The listing builds one solid part. Answer for the finished solid, in the listing's coordinates (mm). Face numbers are marked on the shaded views. A direction names the side the tool comes from. Round coordinates to 2 decimals unless told otherwise and drop trailing zeros. Write each loop counter-clockwise with the first axis right and the second up, starting at its lowest first coordinate (ties: lowest second). Pieces come first, ordered by that corner, then holes. Notation, with made-up numbers: M 3.5,-39 L 13.5,-39 A6 ccw 13.5,-31 Z; hole C 16.5,79 d9. An arc over 180 degrees is marked long. One line per item, written item: value. Start each with the question number.
(1) Given P1, Ø12, axis at x = -8, z = 12.5, coming from the -Y side; P2, Ø9.5, axis at x = 33.26, y = 5, coming from the +Z side; P3, Ø8, axis at x = 27, y = 7.5, coming from the +Z side, each flat-ended and moving along its own axis, determine where each tip first touches the part or whether it passes through.
(2) Section A-A (y = -12.5) is taken. Determine the outline of the cut face in (x, z) (3 decimals), plus the area to 3 significant figures.
(3) Section D-D (z = 16.5) is taken. Determine the outline of the cut face in (x, y) (3 decimals), plus the area to 3 significant figures.
(4) Section B-B (y = 5) is taken. State how many separate pieces and enclosed holes the cut face has, plus the area to 3 significant figures.
(5) Section C-C (x = -9) is taken. Determine the outline of the cut face in (y, z), plus the area to 3 significant figures.
(6) Consider probe 1 along X at (y, z) = (1.5, 6); probe 2 along X at (y, z) = (-21, 4) (3 decimals); probe 3 along Z at (x, y) = (-55, -12.5). Determine where each line is inside the solid, lowest interval first.
(7) For the marked faces 1, 2, 3 and 4, determine the directions among +Z, -Z, +X, -X, +Y, -Y from which every point of the face is accessible in a straight line to the end or side of a thin tool.
(8) For a pull along Z with two mould halves and no side action, classify the marked faces 5, 6 and 7 as released by +Z, released by -Z, zero draft, split by the parting line, or undercut.
Autodesk Inventor part; units mm, degrees
ref_plane "YZ Plane" through (0, 0, 0) normal (1, 0, 0) x (0, 1, 0)
ref_plane "XZ Plane" through (0, 0, 0) normal (0, 1, 0) x (-1, 0, 0)
ref_plane "XY Plane" through (0, 0, 0) normal (0, 0, 1) x (1, 0, 0)
sketch "Sketch1" plane through (0, 0, 0) normal (0, 1, 0) x (-1, 0, 0)
  line L0 (-15, 15) -> (15, 15)
  line L1 (15, 15) -> (15, -15)
  line L2 (15, -15) -> (-15, -15)
  line L3 (-15, 15) -> (15, -15) construction
  line L4 (15, 15) -> (-15, -15) construction
  line L5 (25, 25) -> (-25, 25)
  line L6 (-25, -25) -> (25, -25)
  line L7 (25, 25) -> (59.45, 25)
  line L8 (59.45, 25) -> (59.45, -25)
  line L9 (59.45, -25) -> (25, -25)
  line L10 (-40.9844, -10.0467) -> (-25, -10.0467)
  line L11 (-25, 10.0467) -> (-40.9844, 10.0467)
  line L12 (-40.9844, -10.0467) -> (-20.5822, 10.0467) construction
  line L13 (-27.4388, -3.2939) -> (-40.9844, 10.0467) construction
  line L14 (-40.9844, -3.2939) -> (-15, -3.2939)
  line L15 (-15, 3.2939) -> (-40.9844, 3.2939)
  line L16 (-46.5666, -3.2939) -> (-15, 3.2939) construction
  line L17 (-15, -3.2939) -> (-46.5666, 3.2939) construction
  line L18 (-40.9844, 10.0467) -> (-40.9844, 3.2939)
  line L19 (-40.9844, -3.2939) -> (-40.9844, -10.0467)
  line L20 (-25, 25) -> (-25, 10.0467)
  line L21 (-15, -15) -> (-15, -3.2939)
  line L22 (-15, 3.2939) -> (-15, 15)
  line L23 (-25, -10.0467) -> (-25, -25)
  point P0 (0, 0)
  point P1 (-30.7833, 0)
  dimension "d0" = 30
  dimension "d1" = 30
  dimension "d2" = 10
  dimension "d4" = 44.45
extrude "Extrusion1" add sketch "Sketch1" along normal blind 10
sketch "Sketch2" plane through (0, 0, 0) normal (0, -1, 0) x (1, 0, 0)
  line L0 (15, 15) -> (-15, 15)
  line L1 (15, 3.2939) -> (15, 15)
  line L2 (40.9844, 3.2939) -> (15, 3.2939)
  line L3 (40.9844, 10.0467) -> (40.9844, 3.2939)
  line L4 (25, 10.0467) -> (40.9844, 10.0467)
  line L5 (25, 25) -> (25, 10.0467)
  line L6 (-59.45, 25) -> (25, 25)
  line L7 (-59.45, -25) -> (-59.45, 25)
  line L8 (25, -25) -> (-59.45, -25)
  line L9 (25, -10.0467) -> (25, -25)
  line L10 (40.9844, -10.0467) -> (25, -10.0467)
  line L11 (40.9844, -3.2939) -> (40.9844, -10.0467)
  line L12 (15, -3.2939) -> (40.9844, -3.2939)
  line L13 (15, -15) -> (15, -3.2939)
  line L14 (-15, -15) -> (15, -15)
  line L15 (-15, 15) -> (-15, -15)
  line L16 (-49.725, -25) -> (-24.725, -25)
  line L17 (-24.725, -25) -> (-24.725, 25)
  line L18 (-24.725, 25) -> (-49.725, 25)
  line L19 (-49.725, 25) -> (-49.725, -25)
  line L20 (-49.725, -25) -> (-24.725, 25) construction
  line L21 (-24.725, -25) -> (-49.725, 25) construction
  line L22 (-59.45, 25) -> (25, 25)
  line L23 (-15, 25) -> (-15, -25)
  line L24 (25, -25) -> (-59.45, -25)
  line L25 (-59.45, 25) -> (-49.725, 25)
  line L26 (-59.45, 25) -> (25, 25)
  line L27 (-24.725, 25) -> (-15, 25)
  line L28 (-59.45, 21.5922) -> (-49.725, 21.5922)
  line L29 (-24.725, 21.5922) -> (-15, 21.5922)
  line L30 (-15, 15) -> (-15, -15)
  point P0 (0, 0)
  point P1 (-37.225, 0)
  point P2 (-15, -25)
  dimension "d7" = 25
extrude "Extrusion2" add sketch "Sketch2" along normal blind 25 contours L15 L23 L8 L17 L29 | L29 L17 L6 L23 | L8 L7 L28 L19 | L19 L28 L7 L6
sketch "Sketch3" plane through (-24.725, 0, -25) normal (-1, 0, 0) x (0, 0, 1)
  line L0 (0, 0) -> (50, 0) construction
  line L1 (0, 0) -> (0, -25) construction
  line L2 (50, -25) -> (0, -25) construction
  line L3 (50, 0) -> (50, -25) construction
  line L4 (0, -12.5) -> (50, -12.5) construction
  line L5 (50, 0) -> (50, -25) construction
  line L6 (15, -12.5) -> (35, -12.5) construction
  line L7 (15, -15.2) -> (35, -15.2) construction
  line L8 (35, -9.8) -> (15, -9.8) construction
  arc A0 (15, -9.8) -> (15, -15.2) centre (15, -12.5) ccw construction
  arc A1 (35, -15.2) -> (35, -9.8) centre (35, -12.5) ccw
  circle A2 centre (35, -12.5) radius 2.7
  circle A3 centre (15, -12.5) radius 2.7
  point P0 (25, 0)
  point P1 (25, -12.5)
  point P2 (35, -9.8)
  dimension "d10" = 20
  dimension "d11" = 2.7
extrude "Extrusion3" cut sketch "Sketch3" along normal through all both and the other way through all
fillet "Fillet1" radius 5 10 edges at (-15, 0, 20) (-15, 0, -20) (25, 5, -25) (25, 5, -10.0467) (25, 5, 10.0467) (25, 5, 25) (-19.8625, -25, 25) (-19.8625, -25, -25) (-54.5875, -25, -25) (-54.5875, -25, 25)
sketch "Sketch4" plane through (40.9844, 0, 10.0467) normal (0, 0, 1) x (1, 0, 0)
  line L0 (-10.9844, 0) -> (-10.9844, 10)
  line L1 (-10.9844, 0) -> (0, 0)
  line L2 (0, 0) -> (0, 10)
  line L3 (-10.9844, 10) -> (0, 10)
  circle A0 centre (-7.7256, 5) radius 2
  point P0 (-40.9844, 0)
  dimension "d15" = 4
extrude "Extrusion4" cut sketch "Sketch4" against normal through all contours A0
sketch "Sketch5" plane through (40.9844, 0, 10.0467) normal (0, 0, 1) x (1, 0, 0)
  circle A0 centre (-7.7256, 5) radius 2
  circle A1 centre (-7.7256, 5) radius 3.6921
  point P0 (-40.9844, 0)
extrude "Extrusion5" cut sketch "Sketch5" along normal mid plane 5
properties part number "estopMountV1"
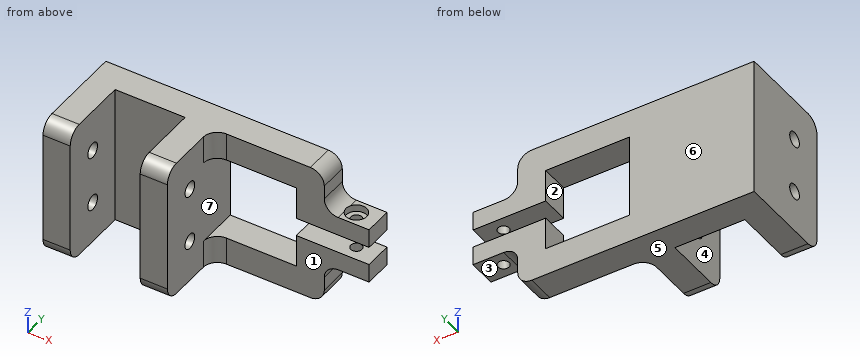
Recorded:
1. P1: stops at y = -1.39
1. P2: stops at z = 10.27
1. P3: stops at z = 24
2. outline: M -59.45,-25 L -49.725,-25 L -49.725,-12.7 L -59.45,-12.7 Z; M -59.45,-7.3 L -49.725,-7.3 L -49.725,7.3 L -59.45,7.3 Z; M -59.45,12.7 L -49.725,12.7 L -49.725,25 L -59.45,25 Z; M -24.725,-25 L -15,-25 L -15,-12.7 L -24.725,-12.7 Z; M -24.725,-7.3 L -15,-7.3 L -15,7.3 L -24.725,7.3 Z; M -24.725,12.7 L -15,12.7 L -15,25 L -24.725,25 Z
2. area: 762 mm2
3. outline: M -59.45,-25 L -49.725,-25 L -49.725,0 L -24.725,0 L -24.725,-25 L -15,-25 L -15,-5 A5 cw -10,0 L 25,0 L 25,10 L -59.45,10 Z
3. area: 1,340 mm2
4. separate pieces: 3
4. enclosed holes: 0
4. area: 3,410 mm2
5. outline: M 0,-25 L 10,-25 L 10,-15 L 0,-15 Z; M 0,15 L 10,15 L 10,25 L 0,25 Z
5. area: 200 mm2
6. probe 1: x = -59.45 to -15, 15 to 40.98
6. probe 2: x = -59.45 to -49.725, -24.725 to -15
6. probe 3: z = -25 to -12.7, -7.3 to 7.3, 12.7 to 25
7. face 1: +Z, -Z, +X, -Y
7. face 2: +Y, -Y
7. face 3: -Z, +X, +Y, -Y
7. face 4: +Z, -Z, -Y
8. face 5: released by -Z
8. face 6: zero draft
8. face 7: undercut
